Print and shaded views of the part. All mm, measured from the part's lowest x, y and z. A direction names the side the tool comes from. Coordinates: 2 decimals unless noted, no trailing zeros. Order: outer loops, then holes, each group sorted by start corner. A loop starts at its lowest first (then second) coordinate and runs counter-clockwise, first axis right, second up. Notation, with made-up numbers: (32.25, 35.5) -> (65.25, 35.5) arc R23 cw to (65.25, 45.5) -> close; hole circle Ø10 at (27.5, 4.25). An arc over 180 degrees is marked (long way). Return JSON: item names as keys, results as strings. Group by question number.
1) Cut at C-C (z = 9). Write the cut outline in (x, y).
2) Cut at B-B (x = 8). Write the cut outline in (y, z).
3) Cut at A-A (y = 8). Write the cut outline in (x, z), and give its area (3 significant figures).
4) Cut at D-D (x = 6.25). Write the cut outline in (y, z), and give its area (3 significant figures).
5) Probe line 1 (Z direction, x = 15, y = 10.5); line 2 (X direction, y = 8, z = 2.5); line 3 (X direction, y = 10, z = 9) (1 decimal). List the from-to ranges inside material, lowest first.
6) Which spindle directions (+Z, -Z, +X, -X, +Y, -Y) get a long thin tool onto all of the face, cutting with end or side? Do the marked faces 1, 2 and 3. Say none if no direction does.
7) Flat gauge pins, fed straight in: pin 1 (3 mm diameter, centred on y = 11, z = 4.5, fed in from -X); pin 2 (2 mm diameter, centred on x = 7, z = 16, fed in from -Y); pin 3 (4 mm diameter, centred on y = 9, z = 9, fed in from +X); pin 4 (1 mm diameter, centred on y = 12.5, z = 18.5, fed in from -X). Where does each tip first touch, or does it go through?
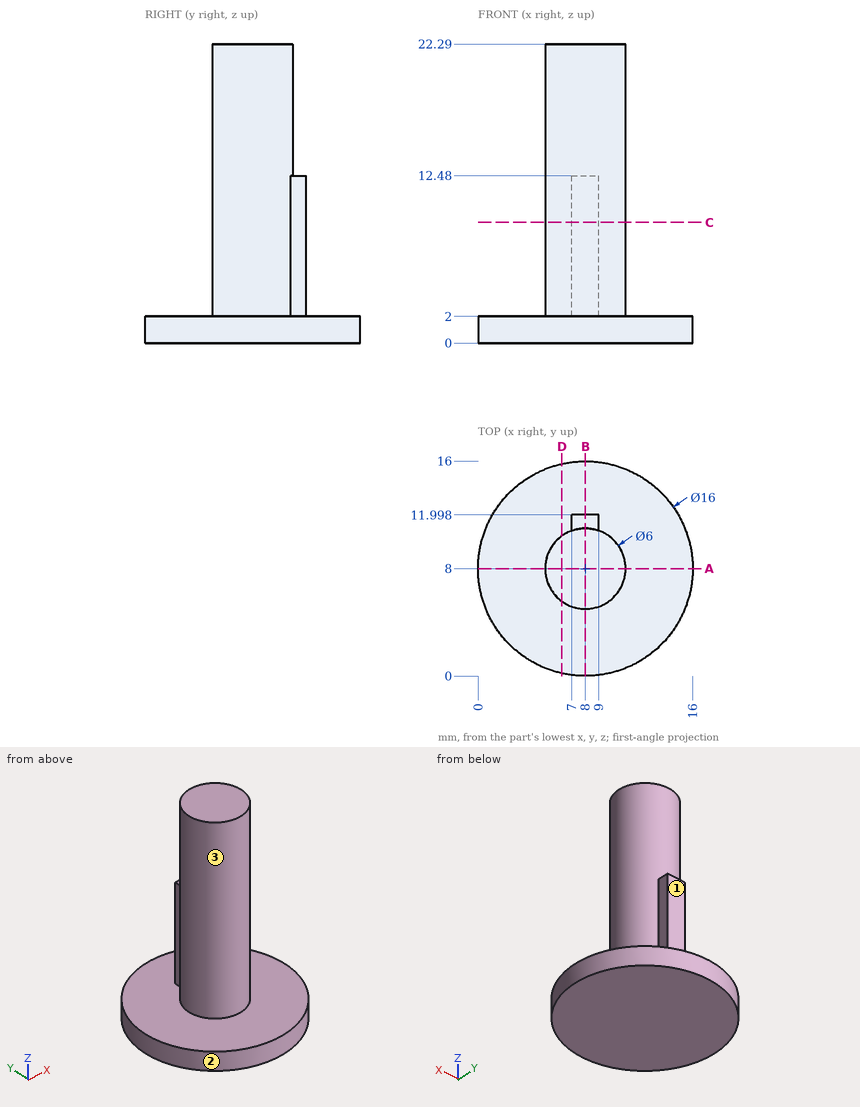
Answers below:
{
 "1": {"outline": "(7, 10.83) arc R3 ccw (long way) to (9, 10.83) -> (9, 12) -> (7, 12) -> close"},
 "2": {"outline": "(0, 0) -> (16, 0) -> (16, 2) -> (12, 2) -> (12, 12.48) -> (11, 12.48) -> (11, 22.29) -> (5, 22.29) -> (5, 2) -> (0, 2) -> close"},
 "3": {"outline": "(0, 0) -> (16, 0) -> (16, 2) -> (11, 2) -> (11, 22.29) -> (5, 22.29) -> (5, 2) -> (0, 2) -> close", "area": "154 mm^2"},
 "4": {"outline": "(0.19, 0) -> (15.81, 0) -> (15.81, 2) -> (10.44, 2) -> (10.44, 22.29) -> (5.56, 22.29) -> (5.56, 2) -> (0.19, 2) -> close", "area": "130 mm^2"},
 "5": {"line 1": "z = 0 to 2", "line 2": "x = 5 to 11", "line 3": "x = 5.8 to 10.2"},
 "6": {"face 1": "+Z, +X, -X, +Y", "face 2": "+Z, -Z", "face 3": "+Z"},
 "7": {"pin 1": "stops at x = 5.4", "pin 2": "stops at y = 5", "pin 3": "stops at x = 11", "pin 4": "passes through"}
}
